```python
from build123d import *

# Parameters (mm, degrees)
BOSS_EXTRUDE1_DEPTH         = 15
SHELL1_T                    = -2
SKETCH3_R                   = 5
CUT_EXTRUDE1_DEPTH          = 110.402425133
BOSS_EXTRUDE2_REACH         = 110.664
SKETCH4_R                   = 3
BOSS_EXTRUDE2_DRAFT         = 1
M3_TAPPED_HOLE1_D           = 2.5
M3_TAPPED_HOLE1_DEPTH       = 6
M3_TAPPED_HOLE1_CSINK_D     = 3.5
M3_TAPPED_HOLE1_CSINK_ANGLE = 90
M3_TAPPED_HOLE1_TIP         = 0.751075774
SKETCH14_R                  = 0.75
CUT_EXTRUDE3_DEPTH          = 10
SKETCH20_R                  = 0.75
CUT_EXTRUDE4_DEPTH          = 10


with BuildPart() as part:
    # Sketch1 → Boss-Extrude1 (new body)
    with BuildSketch(Plane.XY):
        with BuildLine():
            Line((-49, 66.375), (49, 66.375))
            ThreePointArc((49, 66.375), (53.242640687, 64.617640687), (55, 60.375))
            Line((55, 60.375), (55, -87.375))
            ThreePointArc((55, -87.375), (53.242640687, -91.617640687), (49, -93.375))
            Line((49, -93.375), (-49, -93.375))
            ThreePointArc((-49, -93.375), (-53.242640687, -91.617640687), (-55, -87.375))
            Line((-55, -87.375), (-55, 60.375))
            ThreePointArc((-55, 60.375), (-53.242640687, 64.617640687), (-49, 66.375))
        make_face()
    extrude(amount=BOSS_EXTRUDE1_DEPTH)

    # Shell1
    shell1_openings = [part.faces().sort_by_distance(p)[0] for p in [
        (0, -13.5, 0),
    ]]
    offset(amount=SHELL1_T, openings=shell1_openings, kind=Kind.INTERSECTION)

    # Sketch3 → Cut-Extrude1 (cut, through all)
    with BuildSketch(Plane.XY.offset(15)):
        with Locations((-24.5, 3.875)):
            Circle(SKETCH3_R)
        with Locations((24.5, 3.875)):
            Circle(SKETCH3_R)
        with BuildLine():
            Line((-33.45, 47.075), (33.45, 47.075))
            ThreePointArc((33.45, 47.075), (33.803553391, 46.928553391), (33.95, 46.575))
            Line((33.95, 46.575), (33.95, 30.675))
            ThreePointArc((33.95, 30.675), (33.803553391, 30.321446609), (33.45, 30.175))
            Line((33.45, 30.175), (-33.45, 30.175))
            ThreePointArc((-33.45, 30.175), (-33.803553391, 30.321446609), (-33.95, 30.675))
            Line((-33.95, 30.675), (-33.95, 46.575))
            ThreePointArc((-33.95, 46.575), (-33.803553391, 46.928553391), (-33.45, 47.075))
        make_face()
    extrude(amount=-CUT_EXTRUDE1_DEPTH, mode=Mode.SUBTRACT)




with BuildPart() as boss_extrude2_long_prism_1:
    # Sketch4 → Boss-Extrude2 (the long prism of profile 1, to be tilted and cut off)
    with BuildSketch(Plane(origin=(0, 0, 7), x_dir=(-1, 0, 0), z_dir=(0, 0, -1))):
        with Locations((-45, 56.375)):
            Circle(SKETCH4_R)
    extrude(amount=-BOSS_EXTRUDE2_REACH)
    boss_extrude2_tool1_sides = [boss_extrude2_long_prism_1.faces().sort_by_distance(p)[0] for p in [
        (48, 56.375, 62.332),
    ]]
    draft(boss_extrude2_tool1_sides, Plane(origin=(0, 0, 7), x_dir=(-1, 0, 0), z_dir=(0, 0, -1)), BOSS_EXTRUDE2_DRAFT)  # the draft: side faces tilted about the start plane


with BuildPart() as part_1:
    add(part.part)
    boss_extrude2_tool1 = boss_extrude2_long_prism_1.part - part.part



with BuildPart() as boss_extrude2_long_prism_2:
    # Sketch4 → Boss-Extrude2 (the long prism of profile 2, to be tilted and cut off)
    with BuildSketch(Plane(origin=(0, 0, 7), x_dir=(-1, 0, 0), z_dir=(0, 0, -1))):
        with Locations((-45, -56.375)):
            Circle(SKETCH4_R)
    extrude(amount=-BOSS_EXTRUDE2_REACH)
    boss_extrude2_tool2_sides = [boss_extrude2_long_prism_2.faces().sort_by_distance(p)[0] for p in [
        (48, -56.375, 62.332),
    ]]
    draft(boss_extrude2_tool2_sides, Plane(origin=(0, 0, 7), x_dir=(-1, 0, 0), z_dir=(0, 0, -1)), BOSS_EXTRUDE2_DRAFT)  # the draft: side faces tilted about the start plane


with BuildPart() as part_2:
    add(part_1.part)
    boss_extrude2_tool2 = boss_extrude2_long_prism_2.part - part.part



with BuildPart() as boss_extrude2_long_prism_3:
    # Sketch4 → Boss-Extrude2 (the long prism of profile 3, to be tilted and cut off)
    with BuildSketch(Plane(origin=(0, 0, 7), x_dir=(-1, 0, 0), z_dir=(0, 0, -1))):
        with Locations((45, 56.375)):
            Circle(SKETCH4_R)
    extrude(amount=-BOSS_EXTRUDE2_REACH)
    boss_extrude2_tool3_sides = [boss_extrude2_long_prism_3.faces().sort_by_distance(p)[0] for p in [
        (-42, 56.375, 62.332),
    ]]
    draft(boss_extrude2_tool3_sides, Plane(origin=(0, 0, 7), x_dir=(-1, 0, 0), z_dir=(0, 0, -1)), BOSS_EXTRUDE2_DRAFT)  # the draft: side faces tilted about the start plane


with BuildPart() as part_3:
    add(part_2.part)
    boss_extrude2_tool3 = boss_extrude2_long_prism_3.part - part.part



with BuildPart() as boss_extrude2_long_prism_4:
    # Sketch4 → Boss-Extrude2 (the long prism of profile 4, to be tilted and cut off)
    with BuildSketch(Plane(origin=(0, 0, 7), x_dir=(-1, 0, 0), z_dir=(0, 0, -1))):
        with Locations((45, -56.375)):
            Circle(SKETCH4_R)
    extrude(amount=-BOSS_EXTRUDE2_REACH)
    boss_extrude2_tool4_sides = [boss_extrude2_long_prism_4.faces().sort_by_distance(p)[0] for p in [
        (-42, -56.375, 62.332),
    ]]
    draft(boss_extrude2_tool4_sides, Plane(origin=(0, 0, 7), x_dir=(-1, 0, 0), z_dir=(0, 0, -1)), BOSS_EXTRUDE2_DRAFT)  # the draft: side faces tilted about the start plane


with BuildPart() as part_4:
    add(part_3.part)
    boss_extrude2_tool4 = boss_extrude2_long_prism_4.part - part.part
    add(boss_extrude2_tool1.solids().sort_by_distance((45, 56.375, 7))[0])
    add(boss_extrude2_tool2.solids().sort_by_distance((45, -56.375, 7))[0])
    add(boss_extrude2_tool3.solids().sort_by_distance((-45, 56.375, 7))[0])
    add(boss_extrude2_tool4.solids().sort_by_distance((-45, -56.375, 7))[0])

    # M3 Tapped Hole1
    with Locations(Plane(origin=(0, 0, 7), x_dir=(-1, 0, 0), z_dir=(0, 0, -1))):
        with Locations((-45, 56.375), (45, 56.375), (45, -56.375), (-45, -56.375)):
            CounterSinkHole(M3_TAPPED_HOLE1_D / 2, M3_TAPPED_HOLE1_CSINK_D / 2, depth=M3_TAPPED_HOLE1_DEPTH, counter_sink_angle=M3_TAPPED_HOLE1_CSINK_ANGLE)
            with Locations((0, 0, -(M3_TAPPED_HOLE1_DEPTH + M3_TAPPED_HOLE1_TIP / 2))):  # 118° drill point
                Cone(0, M3_TAPPED_HOLE1_D / 2, M3_TAPPED_HOLE1_TIP, mode=Mode.SUBTRACT)

    # Sketch14 → Cut-Extrude3 (cut)
    with BuildSketch(Plane.XY.offset(15)):
        with Locations((0, 6.375)):
            Circle(SKETCH14_R)
        with Locations((0, 1.375)):
            Circle(SKETCH14_R)
        with Locations((2.5, 3.875)):
            Circle(SKETCH14_R)
        with Locations((-2.5, 3.875)):
            Circle(SKETCH14_R)
    extrude(amount=-CUT_EXTRUDE3_DEPTH, mode=Mode.SUBTRACT)

    # Sketch17 → CSK for M3 Countersunk Flat Head Screw1 (revolve, cut)
    with BuildSketch(Plane(origin=(-55, 0, 5), x_dir=(0, 0, 1), z_dir=(0, 1, 0))):
        Polygon((0, 0), (0, 2), (1.7, 2), (1.7, 1.45), (3.15, 0), align=None)
    revolve(axis=Axis((-61.35, 0, 5), (1, 0, 0)), mode=Mode.SUBTRACT)

    # Sketch19 → CSK SLOT for M3 Countersunk Flat Head Screw1 (revolve, cut)
    with BuildSketch(Plane(origin=(55, 0, 5), x_dir=(0, 0, -1), z_dir=(0, 1, 0))):
        Polygon((0, 0), (0, 2), (1.7, 2), (1.7, 1.45), (3.15, 0), align=None)
    revolve(axis=Axis((61.35, 0, 5), (-1, 0, 0)), mode=Mode.SUBTRACT)

    # Sketch20 → Cut-Extrude4 (cut)
    with BuildSketch(Plane.XY.offset(15)):
        with Locations((-39.79, -34.725)):
            Circle(SKETCH20_R)
    extrude(amount=-CUT_EXTRUDE4_DEPTH, mode=Mode.SUBTRACT)


solid = part_4.part
```
Input: part model. Units: mm. Frame: model coordinates. A direction names the side the tool comes from. Coordinates: 2 decimals unless noted, no trailing zeros. Write each loop counter-clockwise with the first axis right and the second up, starting at its lowest first coordinate (ties: lowest second). Pieces come first, ordered by that corner, then holes. Notation, with made-up numbers: (-0.5, 61.25) - (58.5, 61.25) arc R19 ccw to (58.5, 70.25) - close; hole circle Ø8 at (2, 84.25). An arc over 180 degrees is marked (long way). Put each result on its own line as item: value. Start each with the question number.
1) Contact query for flat-ended pins moving along their axis: pin 1 (4 mm diameter, centred on x = -45, y = 56.375, fed in from -Z); pin 2 (1.4 mm diameter, centred on x = -39.79, y = -34.725, fed in from +Z); pin 3 (2.5 mm diameter, centred on x = 0, y = 6.375, fed in from -Z). Output: stop coordinate, or through.
2) Cut plane C-C (x = 15). Return the cut outline in (y, z) (3 decimals), plus the area to 3 significant figures.
3) Reachability of faces 1 (the face through (55, -12, 7)), 2 (the face through (53, -12, 6)) from +Z, -Z, +X, -X, +Y, -Y: full face, straight path, thin tool, end or side. Return the list, or none.
4) Cut plane B-B (y = 45). Return the cut outline in (x, z).
5) Mould query, pull axis X, two halves, no side actions, for faces 3 (the face through (-55, -15, 7)), 4 (the face through (-1, 66.375, 7)), 5 (the face through (1, -91.375, 6)). Classes: pulls with the +X half, pulls with the -X half, needs draft (parallel to the pull), parting line crosses it, or undercut.
6) Ray query, L1, parallel to Y at x = 0, z = 13.8 (3 decimals); L2, parallel to Y at x = -45, z = 11.1 (3 decimals); L3, parallel to Y at x = 38.5, z = 2.25 (3 decimals). Return the intervals inside material, ascending.
7) Cut plane A-A (z = 10.75). State how many separate pieces and enclosed holes the cut face has, plus the area to 3 significant figures.
8) Cut plane D-D (x = -25). Return the cut outline in (y, z) (3 decimals), plus the area to 3 significant figures.
Resolved:
1. pin 1: stops at z = 7
1. pin 2: passes through
1. pin 3: stops at z = 13
2. outline: (-93.375, 0) - (-91.375, 0) - (-91.375, 13) - (30.175, 13) - (30.175, 15) - (-93.375, 15) - close; (47.075, 13) - (64.375, 13) - (64.375, 0) - (66.375, 0) - (66.375, 15) - (47.075, 15) - close
2. area: 338 mm2
3. face 1: +Z, -Z, +X, +Y, -Y
3. face 2: -Z
4. outline: (-55, 0) - (-53, 0) - (-53, 13) - (-33.95, 13) - (-33.95, 15) - (-55, 15) - close; (33.95, 13) - (53, 13) - (53, 0) - (55, 0) - (55, 15) - (33.95, 15) - close
5. face 3: pulls with the -X half
5. face 4: needs draft
5. face 5: undercut
6. L1: y = -93.375 to 0.625, 2.125 to 5.625, 7.125 to 30.175, 47.075 to 66.375
6. L2: y = -93.375 to -91.375, -59.447 to -57.625, -55.125 to -53.303, 53.303 to 55.125, 57.625 to 59.447, 64.375 to 66.375
6. L3: y = -93.375 to -91.375, 64.375 to 66.375
7. separate pieces: 5
7. enclosed holes: 5
7. area: 1,140 mm2
8. outline: (-93.375, 0) - (-91.375, 0) - (-91.375, 13) - (-1.1, 13) - (-1.1, 15) - (-93.375, 15) - close; (8.85, 13) - (30.175, 13) - (30.175, 15) - (8.85, 15) - close; (47.075, 13) - (64.375, 13) - (64.375, 0) - (66.375, 0) - (66.375, 15) - (47.075, 15) - close
8. area: 318 mm2
